Check sheet for the modelled part. Datum: model origin and axes. Units: mm. A direction names the side the tool comes from. Coordinates: 2 decimals unless noted, no trailing zeros. Loops run counter-clockwise (first coordinate to the right, second up) from the corner with the lowest first, then second, coordinate; pieces in that order, holes last. Notation, with made-up numbers: (4.25, 21.25) -> (58.25, 21.25) arc R13 ccw to (58.25, 27.25) -> close; hole circle Ø4 at (24.5, -18). An arc over 180 degrees is marked (long way). Use CSV: the item, a comma, the result in double quotes.
```python
from build123d import *

# Parameters (mm, degrees)
SCHIZZO1_W                   = 20
SCHIZZO1_H                   = 15
ESTRUSIONE_ESTRUSIONE1_DEPTH = 58.2
SCHIZZO2_R                   = 3
TAGLIO_ESTRUSIONE1_DEPTH     = 60.527220664
SCHIZZO3_R                   = 6.75
TAGLIO_ESTRUSIONE2_DEPTH     = 13
SCHIZZO4_R                   = 1.5
TAGLIO_ESTRUSIONE3_DEPTH     = 62.99588696
FORO_FILETTATO_G1_8_1_D      = 8.8
FORO_FILETTATO_G1_8_1_DEPTH  = 12.72
FORO_FILETTATO_G1_8_1_TIP    = 2.643786724


with BuildPart() as part:
    # Schizzo1 → Estrusione-Estrusione1 (new body)
    with BuildSketch(Plane.XY):
        Rectangle(SCHIZZO1_W, SCHIZZO1_H)
    extrude(amount=-ESTRUSIONE_ESTRUSIONE1_DEPTH)

    # Schizzo2 → Taglio-Estrusione1 (cut, through all)
    with BuildSketch(Plane(origin=(0, 0, -58.2), x_dir=(-1, 0, 0), z_dir=(0, 0, -1))):
        Circle(SCHIZZO2_R)
    extrude(amount=-TAGLIO_ESTRUSIONE1_DEPTH, mode=Mode.SUBTRACT)

    # Schizzo3 → Taglio-Estrusione2 (cut)
    with BuildSketch(Plane(origin=(0, 0, -58.2), x_dir=(-1, 0, 0), z_dir=(0, 0, -1))):
        Circle(SCHIZZO3_R)
    extrude(amount=-TAGLIO_ESTRUSIONE2_DEPTH, mode=Mode.SUBTRACT)

    # Schizzo4 → Taglio-Estrusione3 (cut, through all)
    with BuildSketch(Plane(origin=(10, 0, 0), x_dir=(0, 0, -1), z_dir=(1, 0, 0))):
        with Locations((19.1, 5.5)):
            Circle(SCHIZZO4_R)
        with Locations(Location((39.1, 5.5, 0), (0, 0, 180))):
            Circle(SCHIZZO4_R)
    extrude(amount=-TAGLIO_ESTRUSIONE3_DEPTH, mode=Mode.SUBTRACT)

    # Foro filettato G1/8-1
    with Locations(Plane.XY):
        with Locations((0, 0)):
            Hole(FORO_FILETTATO_G1_8_1_D / 2, depth=FORO_FILETTATO_G1_8_1_DEPTH)
            with Locations((0, 0, -(FORO_FILETTATO_G1_8_1_DEPTH + FORO_FILETTATO_G1_8_1_TIP / 2))):  # 118° drill point
                Cone(0, FORO_FILETTATO_G1_8_1_D / 2, FORO_FILETTATO_G1_8_1_TIP, mode=Mode.SUBTRACT)


solid = part.part
```
1) Cross-section at B-B on z = -19.1. Record the boundary of the cut face in (x, y).
Answer below:
outline,"(-10, -7.5) -> (10, -7.5) -> (10, 4) -> (-10, 4) -> close; (-10, 7) -> (10, 7) -> (10, 7.5) -> (-10, 7.5) -> close; hole circle Ø6 at (0, 0)"
2) Thickness scan on line 1 along Y through (x, z) = (0, -27.5); line 2 along X through (y, z) = (0, -15); line 3 along Y through (x, z) = (-5.5, -19.1). Record the ranges inside material, lowest first. Write a range as from..to.
Answer below:
line 1,"y = -7.5..-3, 3..7.5"
line 2,"x = -10..-3, 3..10"
line 3,"y = -7.5..4, 7..7.5"
3) Cross-section at C-C on y = 0. Record the boundary of the cut face in (x, z), and give its area (3 significant figures).
Answer below:
outline,"(-10, -58.2) -> (-6.75, -58.2) -> (-6.75, -45.2) -> (-3, -45.2) -> (-3, -13.56) -> (-4.4, -12.72) -> (-4.4, 0) -> (-10, 0) -> close; (3, -45.2) -> (6.75, -45.2) -> (6.75, -58.2) -> (10, -58.2) -> (10, 0) -> (4.4, 0) -> (4.4, -12.72) -> (3, -13.56) -> close"
area,"681 mm²"
4) Cross-section at D-D on x = 7.5. Record the boundary of the cut face in (y, z).
Answer below:
outline,"(-7.5, -58.2) -> (7.5, -58.2) -> (7.5, 0) -> (-7.5, 0) -> close; hole circle Ø3 at (5.5, -39.1); hole circle Ø3 at (5.5, -19.1)"
5) Cross-section at A-A on x = 0. Record the boundary of the cut face in (y, z), and give its area (3 significant figures).
Answer below:
outline,"(-7.5, -58.2) -> (-6.75, -58.2) -> (-6.75, -45.2) -> (-3, -45.2) -> (-3, -13.56) -> (-4.4, -12.72) -> (-4.4, 0) -> (-7.5, 0) -> close; (3, -45.2) -> (6.75, -45.2) -> (6.75, -58.2) -> (7.5, -58.2) -> (7.5, 0) -> (4.4, 0) -> (4.4, -12.72) -> (3, -13.56) -> close; hole circle Ø3 at (5.5, -39.1); hole circle Ø3 at (5.5, -19.1)"
area,"375 mm²"
6) Go/stop test with flat-tipped pins: pin 1 Ø4 at (y, z) = (5.5, -19.1) entering from -X; pin 2 Ø6 at (x, y) = (-0.5, 3) entering from -Z. Record where each tip stops, or that it passes through.
Answer below:
pin 1,"stops at x = -10"
pin 2,"stops at z = -45.2"
7) Draft check along Y on faces 3 (the flat face through (10, 0, -29)), 4 (the cylindrical face through (0.14, 5.57, -17.6)), 5 (the cylindrical face through (-4.197, 1.322, -6.449)), 6 (the flat face through (0, -7.5, -29)). Enter one of: released by +Y, released by -Y, zero draft, split by the parting line, or undercut.
Answer below:
face 3,"zero draft"
face 4,"undercut"
face 5,"undercut"
face 6,"released by -Y"
8) Access from +Z, -Z, +X, -X, +Y, -Y to the whole of each face (thin tool, end or side, straight path). Record for faces 1 (the cylindrical face through (3, 0, -30)), 2 (the cylindrical face through (1.46, -6.59, -51.79)).
Answer below:
face 1,"+Z, -Z"
face 2,"-Z"
